For this review, take the finished solid that the model builds, in its own axes (mm). A direction names the side the tool comes from. Coordinates: 2 decimals unless noted, no trailing zeros. Order: outer loops, then holes, each group sorted by start corner. A loop starts at its lowest first (then second) coordinate and runs counter-clockwise, first axis right, second up. Notation, with made-up numbers: (-30, -31.5) -> (17, -31.5) arc R27 cw to (17, 0.5) -> close; hole circle Ø11 at (-9, -31). An arc over 180 degrees is marked (long way). Answer as a JSON object with one key per item and string values. Group by question number.
1) Machinability: for faces 1 (the cylindrical face through (43.85, -16.96, 0.99)), 2 (the flat face through (-4, -78, 0)), 3 (the cylindrical face through (45.869, -81.325, 1.507)), which of the approach directions +Z, -Z, +X, -X, +Y, -Y give a long, thin tool a straight path to every point of the face, cutting with its end or side? Answer none if there is none.
2) Add section B-B, the plane y = -21. Write out the cut boundary in (x, z), then the cut area to 3 significant figures.
3) Wall thickness on L1, parallel to Y at x = 24.75, z = 0.95; L2, parallel to X at y = -38.5, z = 0.35; L3, parallel to Y at x = 15, z = 0.65: over which ranges is each line inside the solid? List them lowest first.
4) Add section C-C, the plane z = 0.7. Count the separate pieces of the cut face and the enclosed holes in it, then the cut area to 3 significant figures.
5) Add section A-A, the plane x = -21. Write out the cut boundary in (y, z), then the cut area to 3 significant figures.
6) For pin 1 (3 mm diameter, centred on x = 47.5, y = -80.5, fed in from +Z); pin 2 (1.6 mm diameter, centred on x = 24.75, y = -3, fed in from +Z), all flat-tipped, find the tip position at first contact; note any pin that passes through.
7) Draft analysis for pull direction X (two halves, no side actions). For faces 4 (the flat face through (0, -4, 2)), 5 (the cylindrical face through (31.41, -1.68, 0.99)), state which applies: +X half, -X half, draft (parallel to the pull), parting line (faces both ways), or undercut.
from build123d import *

# Parameters (mm, degrees)
SKETCH1_W                  = 109.5
SKETCH1_H                  = 83
BOSS_EXTRUDE1_DEPTH        = 2
F_3_2_3_2_DIAMETER_HOLE2_D = 3.2
F_2_6_2_6_DIAMETER_HOLE2_D = 2.6
F_2_6_2_6_DIAMETER_HOLE1_D = 2.6
SKETCH9_R                  = 3
CUT_EXTRUDE1_DEPTH         = 1
F_2_7_2_7_DIAMETER_HOLE1_D = 2.7
FILLET1_R                  = 1
FILLET2_R                  = 3


with BuildPart() as part:
    # Sketch1 → Boss-Extrude1 (new body)
    with BuildSketch(Plane.XY):
        with Locations((0, -41.5)):
            Rectangle(SKETCH1_W, SKETCH1_H)
        with BuildLine():
            Line((28.75, -9), (28.75, -13.1))
            ThreePointArc((28.75, -13.1), (29.628679656, -15.221320344), (31.75, -16.1))
            Line((31.75, -16.1), (41.75, -16.1))
            ThreePointArc((41.75, -16.1), (43.871320344, -16.978679656), (44.75, -19.1))
            Line((44.75, -19.1), (44.75, -31.5))
            Line((44.75, -31.5), (48.75, -31.5))
            Line((48.75, -31.5), (48.75, -41.5))
            Line((48.75, -41.5), (48.75, -51.5))
            Line((48.75, -51.5), (44.75, -51.5))
            Line((44.75, -51.5), (44.75, -74))
            ThreePointArc((44.75, -74), (43.871320344, -76.121320344), (41.75, -77))
            Line((41.75, -77), (-41.75, -77))
            ThreePointArc((-41.75, -77), (-43.871320344, -76.121320344), (-44.75, -74))
            Line((-44.75, -74), (-44.75, -9))
            ThreePointArc((-44.75, -9), (-43.871320344, -6.878679656), (-41.75, -6))
            Line((-41.75, -6), (25.75, -6))
            ThreePointArc((25.75, -6), (27.871320344, -6.878679656), (28.75, -9))
        make_face(mode=Mode.SUBTRACT)
    extrude(amount=BOSS_EXTRUDE1_DEPTH)

    # Ø3.2 (3.2) Diameter Hole2 (through all)
    with Locations(Plane.XY.offset(2)):
        with Locations((-48.25, -3.5), (-48.25, -79.5), (48.25, -79.5), (48.25, -3.5)):
            Hole(F_3_2_3_2_DIAMETER_HOLE2_D / 2)

    # Ø2.6 (2.6) Diameter Hole2 (through all)
    with Locations(Plane.XY.offset(2)):
        with Locations((32.65, -11.6)):
            Hole(F_2_6_2_6_DIAMETER_HOLE2_D / 2)

    # Ø2.6 (2.6) Diameter Hole1 (through all)
    with Locations(Plane.XY.offset(2)):
        with Locations((32.65, -2.07)):
            Hole(F_2_6_2_6_DIAMETER_HOLE1_D / 2)

    # Sketch9 → Cut-Extrude1 (cut)
    with BuildSketch(Plane.XY.offset(2)):
        with Locations((-48.25, -3.5)):
            Circle(SKETCH9_R)
        with Locations((48.25, -3.5)):
            Circle(SKETCH9_R)
        with Locations((48.25, -79.5)):
            Circle(SKETCH9_R)
        with Locations((-48.25, -79.5)):
            Circle(SKETCH9_R)
    extrude(amount=-CUT_EXTRUDE1_DEPTH, mode=Mode.SUBTRACT)

    # Ø2.7 (2.7) Diameter Hole1 (through all)
    with Locations(Plane.XY.offset(2)):
        with Locations((-24.75, -3), (24.75, -3), (-24.75, -80), (24.75, -80)):
            Hole(F_2_7_2_7_DIAMETER_HOLE1_D / 2)

    # Fillet1
    fillet1_edges = [part.edges().sort_by_distance(p)[0] for p in [
        (44.75, -51.5, 1),
        (44.75, -31.5, 1),
    ]]
    fillet(fillet1_edges, radius=FILLET1_R)

    # Fillet2
    fillet2_edges = [part.edges().sort_by_distance(p)[0] for p in [
        (48.75, -31.5, 1),
        (48.75, -51.5, 1),
    ]]
    fillet(fillet2_edges, radius=FILLET2_R - 0.0001)  # a hair under: the kernel refuses the full size


solid = part.part
Output values:
{
 "1": {"face 1": "+Z, -Z", "face 2": "-Z, +X, -X, +Y, -Y", "face 3": "+Z"},
 "2": {"outline": "(-54.75, 0) -> (-44.75, 0) -> (-44.75, 2) -> (-54.75, 2) -> close; (44.75, 0) -> (54.75, 0) -> (54.75, 2) -> (44.75, 2) -> close", "area": "40.0 mm²"},
 "3": {"L1": "y = -83 to -81.35, -78.65 to -77, -6 to -4.35, -1.65 to 0", "L2": "x = -54.75 to -44.75, 48.75 to 54.75", "L3": "y = -83 to -77, -6 to 0"},
 "4": {"separate pieces": "1", "enclosed holes": "11", "area": "2,760 mm²"},
 "5": {"outline": "(-83, 0) -> (-77, 0) -> (-77, 2) -> (-83, 2) -> close; (-6, 0) -> (0, 0) -> (0, 2) -> (-6, 2) -> close", "area": "24.0 mm²"},
 "6": {"pin 1": "stops at z = 1", "pin 2": "passes through"},
 "7": {"face 4": "draft", "face 5": "undercut"}
}
